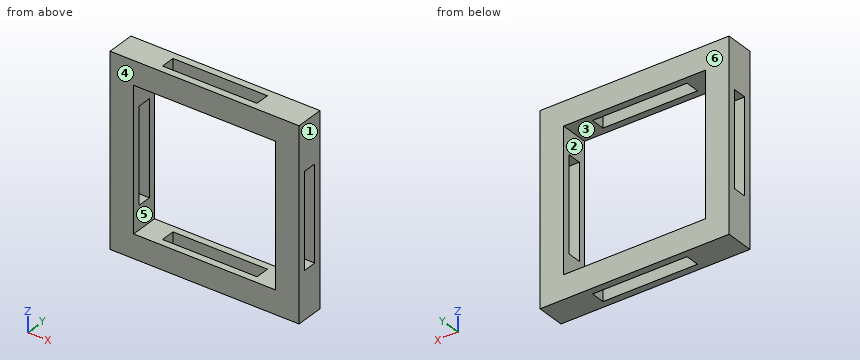
```python
from build123d import *

# Parameters (mm, degrees)
SKETCH1_W           = 20
SKETCH1_H           = 20
SKETCH1_W_2         = 15
SKETCH1_H_2         = 15
BOSS_EXTRUDE1_DEPTH = 3
SKETCH2_W           = 10
SKETCH2_H           = 1.5
CUT_EXTRUDE1_DEPTH  = 21
SKETCH3_W           = 10
SKETCH3_H           = 1.5
CUT_EXTRUDE2_DEPTH  = 21


with BuildPart() as part:
    # Sketch1 → Boss-Extrude1 (new body)
    with BuildSketch(Plane(origin=(0, 0, 0), x_dir=(1, 0, 0), z_dir=(0, 1, 0))):
        Rectangle(SKETCH1_W, SKETCH1_H)
        Rectangle(SKETCH1_W_2, SKETCH1_H_2, mode=Mode.SUBTRACT)
    extrude(amount=BOSS_EXTRUDE1_DEPTH)

    # Sketch2 → Cut-Extrude1 (cut, through all)
    with BuildSketch(Plane.XY.offset(10)):
        with Locations((0, 1.5)):
            Rectangle(SKETCH2_W, SKETCH2_H)
    extrude(amount=-CUT_EXTRUDE1_DEPTH, mode=Mode.SUBTRACT)

    # Sketch3 → Cut-Extrude2 (cut, through all)
    with BuildSketch(Plane.ZY.offset(10)):
        with Locations((0, 1.5)):
            Rectangle(SKETCH3_W, SKETCH3_H)
    extrude(amount=-CUT_EXTRUDE2_DEPTH, mode=Mode.SUBTRACT)


solid = part.part
```
Source: CAD feature listing. Evaluate the final solid. Frame: model axes, mm. Face numbers are marked on the shaded views. A direction names the side the tool comes from. Coordinates: 2 decimals unless noted, no trailing zeros. Loops run counter-clockwise (first coordinate to the right, second up) from the corner with the lowest first, then second, coordinate; pieces in that order, holes last. Notation, with made-up numbers: (-31, 6) -> (25, 6) arc R23 ccw to (25, 41) -> close; hole circle Ø1 at (35, 3). An arc over 180 degrees is marked (long way). One line per item, written item: value. Start each with the question number.
Q1. Section query C-C, the plane x = 3. Return the cut outline in (y, z), and give its area (3 significant figures).
Q2. Section query A-A, the plane z = 5.5. Return the cut outline in (x, y).
Q3. Mould query, pull axis X, two halves, no side actions, for the marked faces 1, 2, 3 and 4. Classes: pulls with the +X half, pulls with the -X half, needs draft (parallel to the pull), parting line crosses it, or undercut.
Q4. Line query: line 1 along X through (y, z) = (2.4, 2); line 2 along Y through (x, z) = (-3.5, -8.5); line 3 along X through (y, z) = (1, -7.75). Output: solid intervals per line, ascending.
Q5. Section query B-B, the plane z = 3. Return the cut outline in (x, y).
Q6. Section query D-D, the plane y = 1.75. Return the cut outline in (x, z).
Q7. Set-up query: the marked faces 5 and 6. Return all of +Z, -Z, +X, -X, +Y, -Y with unobstructed straight access to the full face (end or side cutting, diameter ignored); none if empty.
Results:
1. outline: (0, -10) -> (0.75, -10) -> (0.75, -7.5) -> (0, -7.5) -> close; (0, 7.5) -> (0.75, 7.5) -> (0.75, 10) -> (0, 10) -> close; (2.25, -10) -> (3, -10) -> (3, -7.5) -> (2.25, -7.5) -> close; (2.25, 7.5) -> (3, 7.5) -> (3, 10) -> (2.25, 10) -> close
1. area: 7.50 mm^2
2. outline: (-10, 0) -> (-7.5, 0) -> (-7.5, 3) -> (-10, 3) -> close; (7.5, 0) -> (10, 0) -> (10, 3) -> (7.5, 3) -> close
3. face 1: pulls with the +X half
3. face 2: undercut
3. face 3: undercut
3. face 4: needs draft
4. line 1: -10 to -7.5, 7.5 to 10
4. line 2: 0 to 0.75, 2.25 to 3
4. line 3: -10 to -5, 5 to 10
5. outline: (-10, 0) -> (-7.5, 0) -> (-7.5, 0.75) -> (-10, 0.75) -> close; (-10, 2.25) -> (-7.5, 2.25) -> (-7.5, 3) -> (-10, 3) -> close; (7.5, 0) -> (10, 0) -> (10, 0.75) -> (7.5, 0.75) -> close; (7.5, 2.25) -> (10, 2.25) -> (10, 3) -> (7.5, 3) -> close
6. outline: (-10, -10) -> (-5, -10) -> (-5, -7.5) -> (-7.5, -7.5) -> (-7.5, -5) -> (-10, -5) -> close; (-10, 5) -> (-7.5, 5) -> (-7.5, 7.5) -> (-5, 7.5) -> (-5, 10) -> (-10, 10) -> close; (5, -10) -> (10, -10) -> (10, -5) -> (7.5, -5) -> (7.5, -7.5) -> (5, -7.5) -> close; (5, 7.5) -> (7.5, 7.5) -> (7.5, 5) -> (10, 5) -> (10, 10) -> (5, 10) -> close
7. face 5: +Y, -Y
7. face 6: +Z, -Z, +X, -X, +Y
